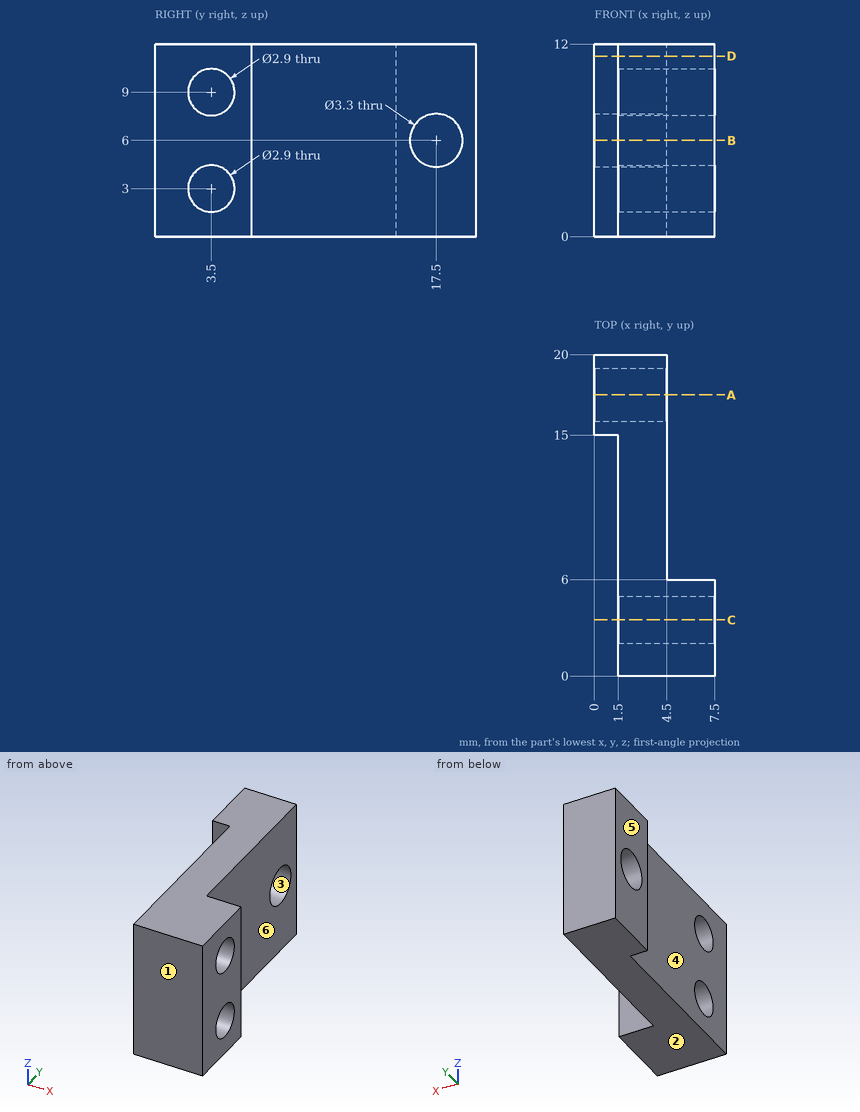
Check sheet for the drawn part. Datum: minimum x, y, z corner. Units: mm. A direction names the side the tool comes from. Coordinates: 2 decimals unless noted, no trailing zeros. Order: outer loops, then holes, each group sorted by start corner. A loop starts at its lowest first (then second) coordinate and runs counter-clockwise, first axis right, second up. Notation, with made-up numbers: (48.25, 24) -> (76.25, 24) arc R20 cw to (76.25, 51) -> close; hole circle Ø4 at (55, 35). An arc over 180 degrees is marked (long way). Use a Markdown table: item, result. Add a question column.
1. Cross-section at C-C (y = 3.5). Enter the section's corners in (x, z), and give its area (3 significant figures).
2. Cross-section at B-B (z = 6). Enter the section's corners in (x, y), and give its area (4 significant figures).
3. Mould release check, pull along Y, two halves, no side actions. Record for the marked faces 1, 2 and 3: pulls with the +Y half, pulls with the -Y half, needs draft (parallel to the pull), parting line crosses it, or undercut.
4. Go/stop test with flat-tipped pins: pin 1 Ø5 at (y, z) = (15, 2) entering from +X; pin 2 Ø1.7 at (y, z) = (3.5, 9) entering from -X; pin 3 Ø0.9 at (x, z) = (5.5, 6) entering from +Y. Record where each tip stops, or that it passes through.
5. Cross-section at D-D (z = 11.25). Enter the section's corners in (x, y).
6. Cross-section at A-A (y = 17.5). Enter the section's corners in (x, z), and give its area (4 significant figures).
7. Material ranges on L1, parallel to X at y = 15.25, z = 5; L2, parallel to X at y = 1.5, z = 9; L3, parallel to Y at x = 5.5, z = 9, recorded low to high.
8. Set-up check for the marked faces 4, 5 and 6: record each of +Z, -Z, +X, -X, +Y, -Y from which the full face is reachable in a straight line by a thin tool's end or side.
Filled sheet:
| question | item | result |
|---|---|---|
| 1 | outline | (1.5, 0) -> (7.5, 0) -> (7.5, 1.55) -> (1.5, 1.55) -> close; (1.5, 4.45) -> (7.5, 4.45) -> (7.5, 7.55) -> (1.5, 7.55) -> close; (1.5, 10.45) -> (7.5, 10.45) -> (7.5, 12) -> (1.5, 12) -> close |
| 1 | area | 37.2 mm2 |
| 2 | outline | (0, 15) -> (1.5, 15) -> (1.5, 0) -> (7.5, 0) -> (7.5, 6) -> (4.5, 6) -> (4.5, 15.85) -> (0, 15.85) -> close; (0, 19.15) -> (4.5, 19.15) -> (4.5, 20) -> (0, 20) -> close |
| 2 | area | 70.65 mm2 |
| 3 | face 1 | pulls with the -Y half |
| 3 | face 2 | needs draft |
| 3 | face 3 | undercut |
| 4 | pin 1 | x = 4.5 |
| 4 | pin 2 | through |
| 4 | pin 3 | y = 6 |
| 5 | outline | (0, 15) -> (1.5, 15) -> (1.5, 0) -> (7.5, 0) -> (7.5, 6) -> (4.5, 6) -> (4.5, 20) -> (0, 20) -> close |
| 6 | outline | (0, 0) -> (4.5, 0) -> (4.5, 4.35) -> (0, 4.35) -> close; (0, 7.65) -> (4.5, 7.65) -> (4.5, 12) -> (0, 12) -> close |
| 6 | area | 39.15 mm2 |
| 7 | L1 | 0 to 4.5 |
| 7 | L2 | 1.5 to 7.5 |
| 7 | L3 | 0 to 2.05, 4.95 to 6 |
| 8 | face 4 | +Z, -Z, -X, -Y |
| 8 | face 5 | +Z, -Z, -X, +Y, -Y |
| 8 | face 6 | +Z, -Z, +X, +Y |
